from build123d import *

# Parameters (mm, degrees)
F0_W     = 76.2
F0_H     = 76.2
F1_DEPTH = 11.938
F3_START = -25.4
F2_R     = 12.7
F2_R_2   = 6.35
F3_DEPTH = 25.4
F4_R     = 6.35
F5_DEPTH = 25.4


with BuildPart() as f1:
    # F0 (on Front) → F1 (new body)
    with BuildSketch(Plane.XZ):
        with Locations((38.1, 38.1)):
            Rectangle(F0_W, F0_H)
    extrude(amount=F1_DEPTH)

    # F2 (on face) → F3 (join)
    with BuildSketch(Plane(origin=(0, 0, 0), x_dir=(0, -1, 0), z_dir=(-1, 0, 0)).offset(F3_START)):
        with Locations((11.5956608206, 82.5315266848)):
            Circle(F2_R)
        with Locations((11.5956608206, 82.5315266848)):
            Circle(F2_R_2, mode=Mode.SUBTRACT)
    extrude(amount=-F3_DEPTH)

    # F4 (on face) → F5 (cut)
    with BuildSketch(Plane.XZ.offset(11.938)):
        with Locations((38.1, 14.7721702233)):
            Circle(F4_R)
        with Locations((17.6816564053, 43.7637194991)):
            Circle(F4_R)
        with Locations((63.2398054004, 43.7637194991)):
            Circle(F4_R)
    extrude(amount=-F5_DEPTH, mode=Mode.SUBTRACT)


solid = f1.part
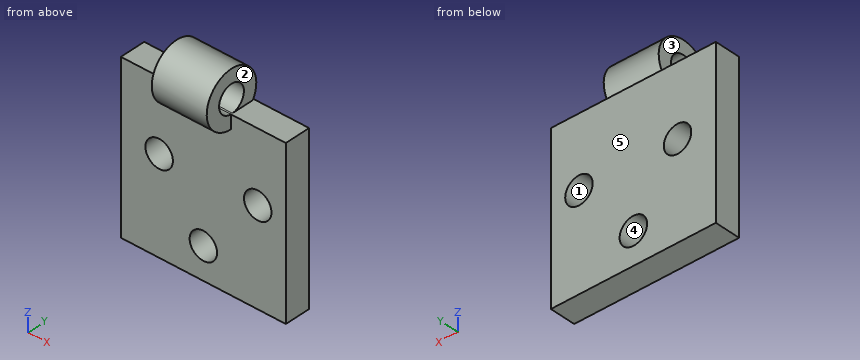
Here's how the part is built. I have some questions about the finished solid (model axes, mm). Face numbers are marked on the shaded views. A direction names the side the tool comes from. Give positions to 0.01 mm unless a question says otherwise; leave off trailing zeros. Order: outer loops, then holes, each group sorted by start corner. A loop starts at its lowest first (then second) coordinate and runs counter-clockwise, first axis right, second up. Notation, with made-up numbers: M -39,29.5 L -21,29.5 A7 cw -21,35.5 Z; hole C 15,38.5 d11. An arc over 180 degrees is marked long. Answer as a JSON object with one key per item and string values. Group by question number.
1) We'd pull the mould along X, two halves only. Please class the marked faces 3, 4 and 5: pulls with the +X half, pulls with the -X half, needs draft (parallel to the pull), parting line crosses it, or undercut.
2) Suppose I cut it at C-C, the plane x = 16.5. Write out the boundary of the cut face in (y, z).
3) Suppose I cut it at B-B, the plane y = -8.5. Write out the boundary of the cut face in (x, z), plus the area to 3 significant figures.
4) Suppose I cut it at A-A, the plane x = 38.1. Count the separate pieces of the cut face and the enclosed holes in it, plus the area to 3 significant figures.
5) Suppose I cut it at D-D, the plane y = -13.75. Write out the boundary of the cut face in (x, z), plus the area to 3 significant figures.
6) On a 3-axis mill with a long thin cutter (end or side, diameter ignored), from which of +Z, -Z, +X, -X, +Y, -Y can I reach the whole of each face in a straight line? I mean the marked faces 1 and 2. Say none if no direction works.
7) I'm going to push flat-ended pins straight in: pin 1 Ø14.5 at (x, z) = (38.1, 14.77) entering from +Y; pin 2 Ø4 at (x, y) = (51.5, -7.5) entering from +Z; pin 3 Ø1.5 at (x, y) = (34, -5.5) entering from +Z. Where does each tip first touch, or does it pass through?
8) Please list where these lines run through material, in increasing order: L1, parallel to Z at x = 38.1, y = -7.75; L2, parallel to X at y = -8, z = 41; L3, parallel to Y at x = 41.5, z = 4.5. Write a range as [from, to].
Results found:
{
 "1": {"face 3": "pulls with the -X half", "face 4": "undercut", "face 5": "needs draft"},
 "2": {"outline": "M -11.94,0 L 0,0 L 0,37.52 L -11.94,37.52 Z; M -11.94,50 L 0,50 L 0,76.2 L -11.94,76.2 Z"},
 "3": {"outline": "M 0,0 L 76.2,0 L 76.2,76.2 L 50.8,76.2 L 50.8,76.99 L 25.4,76.99 L 25.4,76.2 L 0,76.2 Z; M 25.4,88.08 L 50.8,88.08 L 50.8,94.85 L 25.4,94.85 Z; hole C 17.68,43.76 d12.7; hole C 38.1,14.77 d12.7; hole C 63.24,43.76 d12.7", "area": "5,620 mm²"},
 "4": {"separate pieces": "2", "enclosed holes": "1", "area": "1,090 mm²"},
 "5": {"outline": "M 25.4,70.02 L 50.8,70.02 L 50.8,76.56 L 25.4,76.56 Z; M 25.4,88.5 L 50.8,88.5 L 50.8,95.05 L 25.4,95.05 Z", "area": "332 mm²"},
 "6": {"face 1": "+Y, -Y", "face 2": "+Z, +X, -Y"},
 "7": {"pin 1": "y = 0", "pin 2": "z = 95.04", "pin 3": "z = 94.05"},
 "8": {"L1": "[0, 8.42], [21.12, 77.48], [87.58, 94.64]", "L2": "[0, 11.96], [23.4, 57.52], [68.96, 76.2]", "L3": "[-11.94, 0]"}
}
